CAD build for the part. Positions are in the model's coordinates, mm. Face numbers are marked on the shaded views. A direction names the side the tool comes from. Give positions to 0.01 mm unless a question says otherwise; leave off trailing zeros. Order: outer loops, then holes, each group sorted by start corner. A loop starts at its lowest first (then second) coordinate and runs counter-clockwise, first axis right, second up.
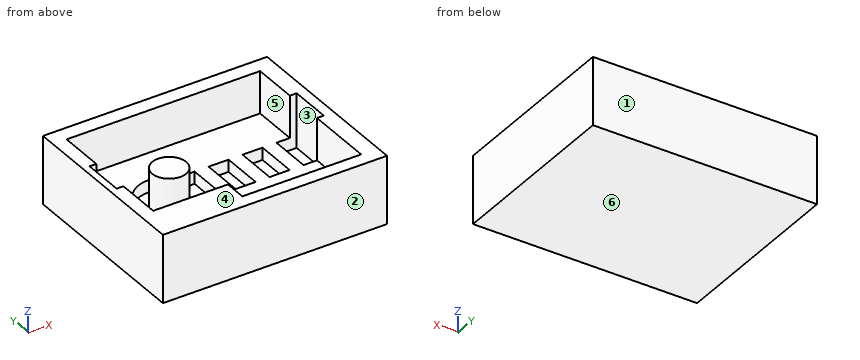
```python
from build123d import *

# Parameters (mm, degrees)
PAD004_DEPTH             = 8.2
SKETCH014_W              = 28.5
SKETCH014_H              = 6.1
PAD005_DEPTH             = 1.8
SKETCH015_R              = 2.9
POCKET004_DEPTH          = 0.6
SKETCH016_W              = 2.05
SKETCH016_H              = 6.1
POCKET005_DEPTH          = 1.8
CLONE012_PLACEMENT_ANGLE = 180
BOX_W                    = 33
BOX_H                    = 27
BOX_DEPTH                = 10
SKETCH_W                 = 3
SKETCH_H                 = 3.25
POCKET009_DEPTH          = 6.2
SKETCH021_W              = 1
SKETCH021_H              = 6.1
POCKET010_DEPTH          = 8
SKETCH022_R              = 4.55
POCKET011_DEPTH          = 1.8
SKETCH023_R              = 2.5
PAD_DEPTH                = 6


with BuildPart() as body011:
    # Sketch013 → Pad004 (new body)
    with BuildSketch(Plane.XY):
        with BuildLine():
            Line((0, 0), (28.5, 0))
            Line((28.5, 0), (28.5, 22.75))
            Line((28.5, 22.75), (14, 22.75))
            Line((14, 22.75), (14, 22.5))
            ThreePointArc((11, 19.5), (13.12132, 20.37868), (14, 22.5))
            Line((11, 19.5), (0, 19.5))
            Line((0, 19.5), (0, 0))
        make_face()
    extrude(amount=PAD004_DEPTH)

    # Sketch014 (on Face9 of Pad004) → Pad005 (join)
    with BuildSketch(Plane.XY.offset(8.2)):
        with Locations((14.25, 9.75)):
            Rectangle(SKETCH014_W, SKETCH014_H)
    extrude(amount=PAD005_DEPTH)

    # Sketch015 (on Face11 of Pad005) → Pocket004 (cut)
    with BuildSketch(Plane.XY.offset(10)):
        with Locations((8.735056, 9.75)):
            Circle(SKETCH015_R)
    extrude(amount=-POCKET004_DEPTH, mode=Mode.SUBTRACT)

    # Sketch016 (on Face10 of Pocket004) → Pocket005 (cut)
    with BuildSketch(Plane.XY.offset(10)):
        with Locations((15.5, 9.75)):
            Rectangle(SKETCH016_W, SKETCH016_H)
        Polygon((21.525, 12.8), (21.525, 6.7), (19.475, 6.7), (19.475, 12.8), (20.5, 12.8), align=None)
        with Locations((25.5, 9.75)):
            Rectangle(SKETCH016_W, SKETCH016_H)
    extrude(amount=-POCKET005_DEPTH, mode=Mode.SUBTRACT)


with BuildPart() as body011_1:
    # Clone012 placement: moved
    add(body011.part.moved(Location((0, 22.75, 12))).rotate(Axis((0, 22.75, 12), (1, 0, 0)), CLONE012_PLACEMENT_ANGLE))


with BuildPart() as model_body012:
    # Box → Box (new body)
    with BuildSketch(Plane(origin=(-2, -2, 0), x_dir=(1, 0, 0), z_dir=(0, 0, 1))):
        with Locations((16.5, 13.5)):
            Rectangle(BOX_W, BOX_H)
    extrude(amount=BOX_DEPTH)

    # Cut: cut Body011
    add(body011_1.part, mode=Mode.SUBTRACT)

    # Sketch (on Face3 of BaseFeature001) → Pocket009 (cut)
    with BuildSketch(Plane.XY.offset(10)):
        with Locations((12.5, 1.625)):
            Rectangle(SKETCH_W, SKETCH_H)
    extrude(amount=-POCKET009_DEPTH, mode=Mode.SUBTRACT)

    # Sketch021 (on Face3 of Pocket009) → Pocket010 (cut)
    with BuildSketch(Plane.XY.offset(10)):
        with Locations((-0.5, 13)):
            Rectangle(SKETCH021_W, SKETCH021_H)
        with Locations((29, 13)):
            Rectangle(SKETCH021_W, SKETCH021_H)
    extrude(amount=-POCKET010_DEPTH, mode=Mode.SUBTRACT)

    # Sketch022 (on Face17 of Pocket010) → Pocket011 (cut)
    with BuildSketch(Plane.XY.offset(3.8)):
        with Locations((8.735056, 13)):
            Circle(SKETCH022_R)
    extrude(amount=-POCKET011_DEPTH, mode=Mode.SUBTRACT)

    # Sketch023 (on Face39 of Pocket011) → Pad (join)
    with BuildSketch(Plane.XY.offset(2)):
        with Locations((8.735056, 13)):
            Circle(SKETCH023_R)
    extrude(amount=PAD_DEPTH)


solid = model_body012.part
```
Item 1: Two-plate mould, pull along Y, no slides. Class the marked faces 1, 2, 3 and 4: released by +Y, released by -Y, zero draft, split by the parting line, or undercut.
Item 2: Slice it at C-C (y = 3.75). Give the cut face in (x, z).
Item 3: Drop flat-ended pins along their axis: pin 1 Ø1.5 at (x, y) = (22.5, 11.5) entering from +Z; pin 2 Ø1 at (x, y) = (25, 1) entering from +Z. Give the stop position or say it passes through.
Item 4: Slice it at D-D (x = 20). Give the cut face in (y, z).
Item 5: Slice it at B-B (z = 9.25). Give the cut face in (x, y).
Item 6: Tool access for the marked faces 5 and 6: list every direction of +Z, -Z, +X, -X, +Y, -Y with a clear straight run to the whole face (end or side of a thin tool).
Item 7: Slice it at A-A (z = 4.75). Give the cut face in (x, y), and give its area (3 significant figures).
Item 8: Wall check: L1, parallel to X at y = 11, z = 9.5; L2, parallel to Y at x = 17.5, z = 3; L3, parallel to Y at x = 9, z = 5. Give the ranges that are in metal, low to high.
A:
1. face 1: released by +Y
1. face 2: released by -Y
1. face 3: undercut
1. face 4: zero draft
2. outline: (-2, 0) - (31, 0) - (31, 10) - (28.5, 10) - (28.5, 3.8) - (0, 3.8) - (0, 10) - (-2, 10) - close
3. pin 1: stops at z = 2
3. pin 2: stops at z = 3.8
4. outline: (-2, 0) - (25, 0) - (25, 10) - (22.75, 10) - (22.75, 3.8) - (0, 3.8) - (0, 10) - (-2, 10) - close
5. outline: (-2, -2) - (31, -2) - (31, 25) - (-2, 25) - close; hole (-1, 9.95) - (0, 9.95) - (0, 3.25) - (11, 3.25) - (11, 0) - (28.5, 0) - (28.5, 9.95) - (29.5, 9.95) - (29.5, 16.05) - (28.5, 16.05) - (28.5, 22.75) - (0, 22.75) - (0, 16.05) - (-1, 16.05) - close
6. face 5: +Z
6. face 6: -Z, +X, -X, +Y, -Y
7. outline: (-2, -2) - (31, -2) - (31, 25) - (-2, 25) - close; circle Ø5 at (8.74, 13); hole (-1, 9.95) - (0, 9.95) - (0, 3.25) - (11, 3.25) - (11, 0) - (28.5, 0) - (28.5, 9.95) - (29.5, 9.95) - (29.5, 16.05) - (28.5, 16.05) - (28.5, 22.75) - (0, 22.75) - (0, 16.05) - (-1, 16.05) - close
7. area: 286 mm2
8. L1: x = -2 to -1, 29.5 to 31
8. L2: y = -2 to 9.95, 16.05 to 25
8. L3: y = -2 to 3.25, 10.51 to 15.49, 22.75 to 25
